Read the model definition and answer for the solid it produces. Units are mm, in the model's axes. Face numbers are marked on the shaded views. A direction names the side the tool comes from. Round coordinates to 2 decimals unless told otherwise and drop trailing zeros. Loops run counter-clockwise (first coordinate to the right, second up) from the corner with the lowest first, then second, coordinate; pieces in that order, holes last. Notation, with made-up numbers: (22, -10) - (81, -10) arc R31 ccw to (81, 25) - close; hole circle Ø6 at (41.5, -7). An arc over 180 degrees is marked (long way). Answer as CSV lines item,"result".
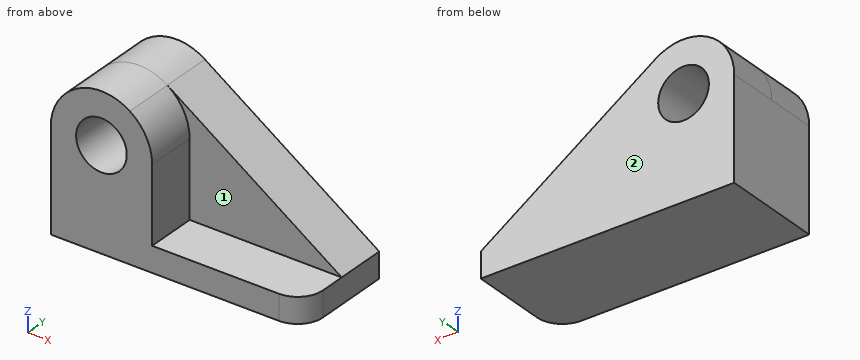
```python
from build123d import *

# Parameters (mm, degrees)
F0_R     = 12.7
F1_DEPTH = 25.4
F3_DEPTH = 25.4
F4_DEPTH = 25.4
F5_R     = 12.7


with BuildPart() as f1:
    # F0 (on Front) → F1 (new body)
    with BuildSketch(Plane.XZ):
        with BuildLine():
            Line((60.523228, -42.777247), (-26.838899, 16.357082))
            ThreePointArc((-26.838899, 16.357082), (-52.983031, 17.759353), (-66.476772, -4.677247))
            Line((-66.476772, -4.677247), (-66.476772, -55.477247))
            Line((-66.476772, -55.477247), (60.523228, -55.477247))
            Line((60.523228, -55.477247), (60.523228, -42.777247))
        make_face()
        with Locations((-41.076772, -4.677247)):
            Circle(F0_R, mode=Mode.SUBTRACT)
    extrude(amount=F1_DEPTH)

    # F2 (on face) → F3 (join)
    with BuildSketch(Plane.XZ.offset(25.4)):
        with BuildLine():
            Line((-15.676772, -4.677247), (-28.376772, -4.677247))
            ThreePointArc((-28.376772, -4.677247), (-41.076772, -17.377247), (-53.776772, -4.677247))
            Line((-53.776772, -4.677247), (-66.476772, -4.677247))
            ThreePointArc((-66.476772, -4.677247), (-41.076772, -30.077247), (-15.676772, -4.677247))
        make_face()
        with BuildLine():
            ThreePointArc((-53.776772, -4.677247), (-41.076772, 8.022753), (-28.376772, -4.677247))
            Line((-28.376772, -4.677247), (-15.676772, -4.677247))
            ThreePointArc((-15.676772, -4.677247), (-41.076772, 20.722753), (-66.476772, -4.677247))
            Line((-66.476772, -4.677247), (-53.776772, -4.677247))
        make_face()
    extrude(amount=F3_DEPTH)

    # F2 (on face) → F4 (join)
    with BuildSketch(Plane.XZ.offset(25.4)):
        with BuildLine():
            Line((-15.676772, -4.677247), (-28.376772, -4.677247))
            ThreePointArc((-28.376772, -4.677247), (-41.076772, -17.377247), (-53.776772, -4.677247))
            Line((-53.776772, -4.677247), (-66.476772, -4.677247))
            ThreePointArc((-66.476772, -4.677247), (-41.076772, -30.077247), (-15.676772, -4.677247))
        make_face()
        with BuildLine():
            ThreePointArc((-53.776772, -4.677247), (-41.076772, 8.022753), (-28.376772, -4.677247))
            Line((-28.376772, -4.677247), (-15.676772, -4.677247))
            ThreePointArc((-15.676772, -4.677247), (-18.640173, 7.229013), (-26.838899, 16.357082))
            ThreePointArc((-26.838899, 16.357082), (-52.983031, 17.759353), (-66.476772, -4.677247))
            Line((-66.476772, -4.677247), (-53.776772, -4.677247))
        make_face()
        with BuildLine():
            Line((-15.676772, -42.777247), (-15.676772, -4.677247))
            ThreePointArc((-15.676772, -4.677247), (-41.076772, -30.077247), (-66.476772, -4.677247))
            Line((-66.476772, -4.677247), (-66.476772, -42.777247))
            Line((-66.476772, -42.777247), (-66.476772, -55.477247))
            Line((-66.476772, -55.477247), (60.523228, -55.477247))
            Line((60.523228, -55.477247), (60.523228, -42.777247))
            Line((60.523228, -42.777247), (-15.676772, -42.777247))
        make_face()
    extrude(amount=F4_DEPTH)

    # F5
    f5_edges = [f1.edges().sort_by_distance(p)[0] for p in [
        (60.523228, -50.8, -49.127247),
    ]]
    fillet(f5_edges, radius=F5_R)


solid = f1.part
```
1) A cutting plane is placed at C-C, the plane x = 51.5. Determine the outline of the cut face in (y, z), plus the area to 3 significant figures.
Entries:
outline,"(-50.26, -55.48) - (0, -55.48) - (0, -36.67) - (-25.4, -36.67) - (-25.4, -42.78) - (-50.26, -42.78) - close"
area,"793 mm^2"
2) A cutting plane is placed at B-B, the plane z = 5.5. Determine the outline of the cut face in (x, y).
Entries:
outline,"(-64.35, -50.8) - (-48.67, -50.8) - (-48.67, 0) - (-64.35, 0) - close; (-33.48, -50.8) - (-17.8, -50.8) - (-17.8, -25.4) - (-10.8, -25.4) - (-10.8, 0) - (-33.48, 0) - close"
3) Find the intervals of material crossed by line 1 (X direction, y = -27, z = -27); line 2 (Z direction, x = 23, y = -44); line 3 (Z direction, x = -44, y = -47), in increasing order.
Entries:
line 1,"x = -66.48 to -15.68"
line 2,"z = -55.48 to -42.78"
line 3,"z = -55.48 to -17.04, 7.68 to 20.55"
4) A cutting plane is placed at D-D, the plane y = -23. Determine the outline of the cut face in (x, z), plus the area to 3 significant figures.
Entries:
outline,"(-66.48, -55.48) - (60.52, -55.48) - (60.52, -42.78) - (-26.84, 16.36) arc R25.4 ccw to (-66.48, -4.68) - close; hole circle Ø25.4 at (-41.08, -4.68)"
area,"6,050 mm^2"
5) A tool of negligible diameter and unlimited length cuts with its end or side. For the marked faces 1 and 2, from which of +Z, -Z, +X, -X, +Y, -Y can it reach the whole face along a straight path? Write none if from no direction.
Entries:
face 1,"+Z, +X, -Y"
face 2,"+Z, -Z, +X, -X, +Y"
6) Each of these flat-tipped pins is pushed along its axis until it touches: P1, Ø12.5, axis at y = -33, z = -20, coming from the +X side; P2, Ø2, axis at x = -29.5, y = -17.5, coming from the +Z side; P3, Ø17.5, axis at x = 30.5, z = -16, coming from the -Y side; P4, Ø1.5, axis at x = 27, z = -21, coming from the +Y side. Where does it stop, or does it pass through?
Entries:
P1,"stops at x = -15.68"
P2,"stops at z = 18.42"
P3,"stops at y = -25.4"
P4,"stops at y = 0"
7) A cutting plane is placed at A-A, the plane y = -34.5. Determine the outline of the cut face in (x, z).
Entries:
outline,"(-66.48, -55.48) - (60.52, -55.48) - (60.52, -42.78) - (-15.68, -42.78) - (-15.68, -4.68) arc R25.4 ccw to (-26.84, 16.36) arc R25.4 ccw to (-66.48, -4.68) - close; hole circle Ø25.4 at (-41.08, -4.68)"
